Geometry check sheet. Reference: drawing and pictorial views, mm from the part's lowest x, y, z. Give positions to 0.01 mm unless a question says otherwise; leave off trailing zeros. Order: outer loops, then holes, each group sorted by start corner. A loop starts at its lowest first (then second) coordinate and runs counter-clockwise, first axis right, second up. Notation, with made-up numbers: (79.25, 52.5) -> (98.25, 52.5) arc R25 cw to (98.25, 68.5) -> close; hole circle Ø6 at (10, -29). An arc over 180 degrees is marked (long way). Write each question's results on one line, items separated by ' | '. Start each with the question number.
1. Material ranges on L1, parallel to Z at x = 20, y = 6, recorded low to high. Write a range as from..to.
2. Depth check by flat-ended pin: pin 1 Ø3 at (x, y) = (13.5, 10) entering from -Z. Enter the tip coordinate at first touch or a pass-through.
3. Mould release check, pull along X, two halves, no side actions. Record for the marked faces 1, 2 and 3: +X half, -X half, draft (parallel to the pull), parting line (faces both ways), or undercut.
4. Cross-section at A-A, the plane x = 0.5. Enter the section's corners in (y, z), then the cut area to 3 significant figures.
5. Cross-section at C-C, the plane x = 24. Enter the section's corners in (y, z).
6. Cross-section at B-B, the plane y = 1.5. Enter the section's corners in (x, z), then the cut area to 3 significant figures.
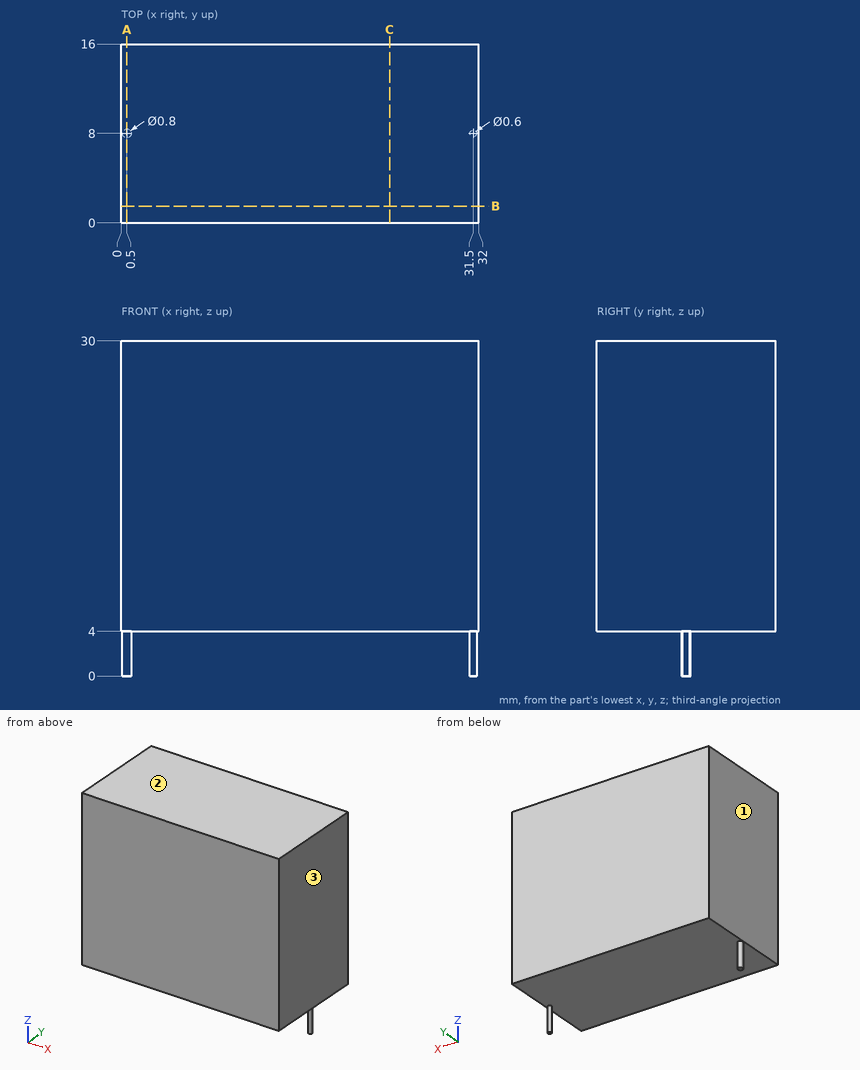
Results below:
1) L1: z = 4..30
2) pin 1: stops at z = 4
3) face 1: -X half | face 2: draft | face 3: +X half
4) outline: (0, 4) -> (7.6, 4) -> (7.6, 0) -> (8.4, 0) -> (8.4, 4) -> (16, 4) -> (16, 30) -> (0, 30) -> close | area: 419 mm²
5) outline: (0, 4) -> (16, 4) -> (16, 30) -> (0, 30) -> close
6) outline: (0, 4) -> (32, 4) -> (32, 30) -> (0, 30) -> close | area: 832 mm²
